from build123d import *

# Parameters (mm, degrees)
SKETCH3_W           = 100
SKETCH3_H           = 50
BOSS_EXTRUDE1_DEPTH = 25
SKETCH5_R           = 8
SKETCH5_W           = 43.746020772
SKETCH5_H           = 23.175190528
CUT_EXTRUDE1_DEPTH  = 76
SKETCH7_R           = 2.5
CUT_EXTRUDE4_DEPTH  = 10
BOSS_EXTRUDE2_START = 10
SKETCH8_W           = 100
SKETCH8_H           = 50
SKETCH8_R           = 2.5
BOSS_EXTRUDE2_DEPTH = 10
SKETCH9_R           = 2.5
CUT_EXTRUDE5_DEPTH  = 10


with BuildPart() as part:
    # Sketch3 → Boss-Extrude1 (new body)
    with BuildSketch(Plane.XY):
        Rectangle(SKETCH3_W, SKETCH3_H)
    extrude(amount=BOSS_EXTRUDE1_DEPTH)

    # Sketch5 → Cut-Extrude1 (cut, through all)
    with BuildSketch(Plane(origin=(0, 25, 0), x_dir=(1, 0, 0), z_dir=(0, 1, 0))):
        with Locations(Location((37, -12.5, 0), (0, 0, 270))):
            Circle(SKETCH5_R)
        with Locations(Location((-37, -12.5, 0), (0, 0, 90))):
            Circle(SKETCH5_R)
        with Locations((0, -13.412404736)):
            Rectangle(SKETCH5_W, SKETCH5_H)
    extrude(amount=-CUT_EXTRUDE1_DEPTH, mode=Mode.SUBTRACT)

    # Sketch7 → Cut-Extrude4 (cut)
    with BuildSketch(Plane(origin=(0, 0, 0), x_dir=(-1, 0, 0), z_dir=(0, 0, -1))):
        with Locations((32.5, 9.25)):
            Circle(SKETCH7_R)
        with Locations((32.5, -9.25)):
            Circle(SKETCH7_R)
        with Locations((-32.5, -9.25)):
            Circle(SKETCH7_R)
        with Locations((-32.5, 9.25)):
            Circle(SKETCH7_R)
    extrude(amount=-CUT_EXTRUDE4_DEPTH, mode=Mode.SUBTRACT)

    # Sketch8 → Boss-Extrude2 (add)
    with BuildSketch(Plane(origin=(0, 0, 0), x_dir=(-1, 0, 0), z_dir=(0, 0, -1)).offset(BOSS_EXTRUDE2_START)):
        Rectangle(SKETCH8_W, SKETCH8_H)
        with Locations((-32.5, 9.25)):
            Circle(SKETCH8_R, mode=Mode.SUBTRACT)
        with Locations((-32.5, -9.25)):
            Circle(SKETCH8_R, mode=Mode.SUBTRACT)
        with Locations((32.5, -9.25)):
            Circle(SKETCH8_R, mode=Mode.SUBTRACT)
        with Locations((32.5, 9.25)):
            Circle(SKETCH8_R, mode=Mode.SUBTRACT)
    extrude(amount=-BOSS_EXTRUDE2_DEPTH)

    # Sketch9 → Cut-Extrude5 (cut)
    with BuildSketch(Plane.XY.offset(1.824809472)):
        with Locations((-15.68, 0)):
            Circle(SKETCH9_R)
        with Locations(Location((15.68, 0, 0), (0, 0, 180))):
            Circle(SKETCH9_R)
    extrude(amount=-CUT_EXTRUDE5_DEPTH, mode=Mode.SUBTRACT)


solid = part.part
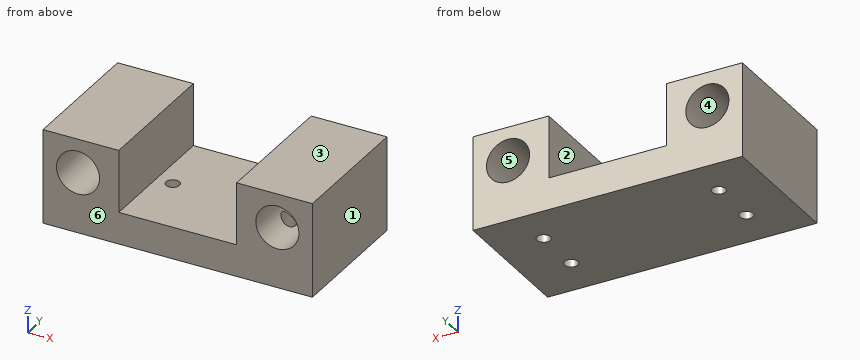
Geometry: final body of the model. Coordinates: model frame, mm. Face numbers are marked on the shaded views. A direction names the side the tool comes from. Give positions to 0.01 mm unless a question says otherwise; leave off trailing zeros. Order: outer loops, then holes, each group sorted by start corner. A loop starts at its lowest first (then second) coordinate and runs counter-clockwise, first axis right, second up. Notation, with made-up numbers: (59, 6) -> (110, 6) arc R21 ccw to (110, 33) -> close; hole circle Ø10 at (-8, 29.25). An arc over 180 degrees is marked (long way). Put each result on its own line as item: value.
Q1. Section A-A, the plane x = -37. Return loops of the section in (y, z).
Here are the results:
outline: (-25, -10) -> (25, -10) -> (25, 4.5) -> (-25, 4.5) -> close; (-25, 20.5) -> (25, 20.5) -> (25, 25) -> (-25, 25) -> close
Q2. Section B-B, the plane z = -6. Return loops of the section in (x, y).
Here are the results:
outline: (-50, -25) -> (50, -25) -> (50, 25) -> (-50, 25) -> close; hole circle Ø5 at (-32.5, -9.25); hole circle Ø5 at (-32.5, 9.25); hole circle Ø5 at (-15.68, 0); hole circle Ø5 at (15.68, 0); hole circle Ø5 at (32.5, -9.25); hole circle Ø5 at (32.5, 9.25)
Q3. Material intervals for L1, parallel to X at y = 12, z = 12; L2, parallel to X at y = 9.25, z = -0.5; L3, parallel to Y at x = -15.5, z = -2, sorted ascending.
Here are the results:
L1: x = -50 to -44.98, -29.02 to -21.87, 21.87 to 29.02, 44.98 to 50
L2: x = -50 to -35, -30 to 30, 35 to 50
L3: y = -25 to -2.49, 2.49 to 25
Q4. Section C-C, the plane y = 5. Return loops of the section in (x, z), then the cut area to 3 significant figures.
Here are the results:
outline: (-50, -10) -> (50, -10) -> (50, 25) -> (21.87, 25) -> (21.87, 1.82) -> (-21.87, 1.82) -> (-21.87, 25) -> (-50, 25) -> close; hole circle Ø16 at (-37, 12.5); hole circle Ø16 at (37, 12.5)
area: 2,080 mm^2
Q5. Reachability of the marked faces 1 and 2 from +Z, -Z, +X, -X, +Y, -Y: full face, straight path, thin tool, end or side. Return the list, or none.
Here are the results:
face 1: +Z, -Z, +X, +Y, -Y
face 2: +Z, +Y, -Y
Q6. Draft query along Z for the marked faces 3, 4, 5 and 6. Return one class per face: released by +Z, released by -Z, zero draft, split by the parting line, or undercut.
Here are the results:
face 3: released by +Z
face 4: undercut
face 5: undercut
face 6: zero draft
Q7. Section D-D, the plane z = 10. Return loops of the section in (x, y), then the cut area to 3 significant figures.
Here are the results:
outline: (-50, -25) -> (-44.6, -25) -> (-44.6, 25) -> (-50, 25) -> close; (-29.4, -25) -> (-21.87, -25) -> (-21.87, 25) -> (-29.4, 25) -> close; (21.87, -25) -> (29.4, -25) -> (29.4, 25) -> (21.87, 25) -> close; (44.6, -25) -> (50, -25) -> (50, 25) -> (44.6, 25) -> close
area: 1,290 mm^2
Q8. Pin query (flat end, axial travel): pin 1 (4.5 mm diameter, centred on x = 15.68, y = 0, fed in from +Z); pin 2 (4.5 mm diameter, centred on x = 32.5, y = 9.25, fed in from -Z); pin 3 (6.5 mm diameter, centred on x = -15.68, y = 0, fed in from +Z). Return the tip coordinate at first contact, or that it passes through.
Here are the results:
pin 1: stops at z = -8.18
pin 2: stops at z = 16.79
pin 3: stops at z = 1.82
